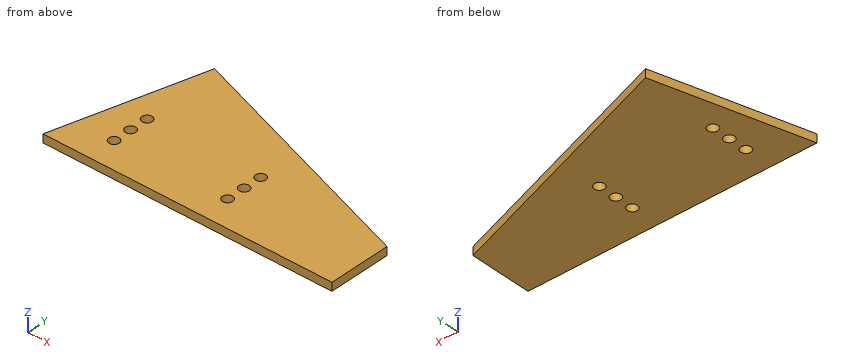
from build123d import *

# Parameters (mm, degrees)
BOSS_EXTRUDE1_DEPTH = 4
SKETCH2_R           = 2.5
CUT_EXTRUDE1_DEPTH  = 10


with BuildPart() as part:
    # Sketch1 → Boss-Extrude1 (new body)
    with BuildSketch(Plane.XY):
        Polygon((75.421686747, -40), (75.421686747, -10), (-45.337786669, 31.806622775), (-64.578313253, -40), align=None)
    extrude(amount=BOSS_EXTRUDE1_DEPTH)

    # Sketch2 → Cut-Extrude1 (cut)
    with BuildSketch(Plane.XY.offset(4)):
        with Locations((-42.578313253, -17)):
            Circle(SKETCH2_R)
        with Locations((-42.578313253, -8)):
            Circle(SKETCH2_R)
        with Locations((-42.578313253, -26)):
            Circle(SKETCH2_R)
        with Locations((12.421686747, -17)):
            Circle(SKETCH2_R)
        with Locations((12.421686747, -8)):
            Circle(SKETCH2_R)
        with Locations((12.421686747, -26)):
            Circle(SKETCH2_R)
    extrude(amount=-CUT_EXTRUDE1_DEPTH, mode=Mode.SUBTRACT)


solid = part.part
Geometry: final body of the model. Coordinates: model frame, mm. Round coordinates to 2 decimals unless told otherwise and drop trailing zeros. Loops run counter-clockwise (first coordinate to the right, second up) from the corner with the lowest first, then second, coordinate; pieces in that order, holes last. Notation, with made-up numbers: (45.5, 13) -> (89.5, 13) arc R18 cw to (89.5, 24) -> close; hole circle Ø5 at (-31.5, -18.5). An arc over 180 degrees is marked (long way). One line per question, with ' | ' between items. Start each with the question number.
1. Section D-D on x = -34.5. Output: boundary loops of the cut face in (y, z), and give its area (3 significant figures).
2. Section B-B on y = -26. Output: boundary loops of the cut face in (x, z), and give its area (3 significant figures).
3. Section A-A on y = -8. Output: boundary loops of the cut face in (x, z), and give its area (3 significant figures).
4. Section C-C on x = 17. Output: boundary loops of the cut face in (y, z).
5. Contact query for a flat-ended pin moving along its axis: pin 1 (3 mm diameter, centred on x = 12.42, y = -8, fed in from +Z). Output: stop coordinate, or through.
6. Line query: line 1 along Y through (x, z) = (11, 0.65); line 2 along Y through (x, z) = (-43, 2.95); line 3 along X through (y, z) = (-16.5, 2.65). Output: solid intervals per line, ascending. Write a range as [from, to].
Returned:
1) outline: (-40, 0) -> (28.05, 0) -> (28.05, 4) -> (-40, 4) -> close | area: 272 mm2
2) outline: (-60.83, 0) -> (-45.08, 0) -> (-45.08, 4) -> (-60.83, 4) -> close; (-40.08, 0) -> (9.92, 0) -> (9.92, 4) -> (-40.08, 4) -> close; (14.92, 0) -> (75.42, 0) -> (75.42, 4) -> (14.92, 4) -> close | area: 505 mm2
3) outline: (-56, 0) -> (-45.08, 0) -> (-45.08, 4) -> (-56, 4) -> close; (-40.08, 0) -> (9.92, 0) -> (9.92, 4) -> (-40.08, 4) -> close; (14.92, 0) -> (69.64, 0) -> (69.64, 4) -> (14.92, 4) -> close | area: 463 mm2
4) outline: (-40, 0) -> (10.23, 0) -> (10.23, 4) -> (-40, 4) -> close
5) pin 1: passes through
6) line 1: y = [-40, -28.06], [-23.94, -19.06], [-14.94, -10.06], [-5.94, 12.3] | line 2: y = [-40, -28.46], [-23.54, -19.46], [-14.54, -10.46], [-5.54, 31] | line 3: x = [-58.28, -45.03], [-40.13, 9.97], [14.87, 75.42]
